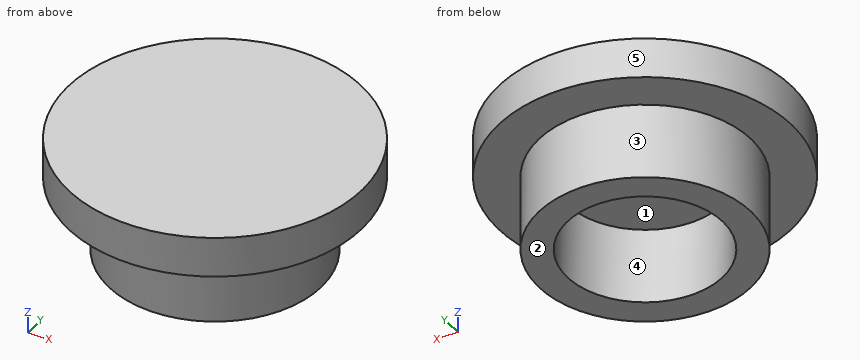
from build123d import *

# Parameters (mm, degrees)
SKETCH1_R           = 9.2075
BOSS_EXTRUDE1_DEPTH = 2.54
SKETCH2_R           = 6.6675
SKETCH2_R_2         = 4.8895
BOSS_EXTRUDE2_DEPTH = 4.7625


with BuildPart() as part:
    # Sketch1 → Boss-Extrude1 (new body)
    with BuildSketch(Plane.XY):
        Circle(SKETCH1_R)
    extrude(amount=BOSS_EXTRUDE1_DEPTH)

    # Sketch2 → Boss-Extrude2 (add)
    with BuildSketch(Plane(origin=(0, 0, 0), x_dir=(-1, 0, 0), z_dir=(0, 0, -1))):
        Circle(SKETCH2_R)
        Circle(SKETCH2_R_2, mode=Mode.SUBTRACT)
    extrude(amount=BOSS_EXTRUDE2_DEPTH)


solid = part.part
Build history of the part. All positions in model axes, mm. Face numbers are marked on the shaded views. A direction names the side the tool comes from. Round coordinates to 2 decimals unless told otherwise and drop trailing zeros. Write each loop counter-clockwise with the first axis right and the second up, starting at its lowest first coordinate (ties: lowest second). Pieces come first, ordered by that corner, then holes. Notation, with made-up numbers: M -26.5,15 L 16.5,15 A8 cw 16.5,19 Z; hole C 74.25,27.5 d4. An arc over 180 degrees is marked long. Answer in a Markdown table with one row per item.
1. Which spindle directions (+Z, -Z, +X, -X, +Y, -Y) get a long thin tool onto all of the face, cutting with end or side? Do the marked faces 4 and 5. Say none if no direction does.
Geometry check:
| item | result |
|---|---|
| face 4 | -Z |
| face 5 | +Z, -Z |
2. Saw through at C-C (y = 3). List the corners of the cut face in (x, z).
Geometry check:
| item | result |
|---|---|
| outline | M -8.71,0 L -5.95,0 L -5.95,-4.76 L -3.86,-4.76 L -3.86,0 L 3.86,0 L 3.86,-4.76 L 5.95,-4.76 L 5.95,0 L 8.71,0 L 8.71,2.54 L -8.71,2.54 Z |
3. Saw through at D-D (z = 1.5). List the corners of the cut face in (x, y) (1 decimal), and give its area (3 significant figures).
Geometry check:
| item | result |
|---|---|
| outline | C 0,0 d18.4 |
| area | 266 mm2 |
4. Mould opens along X. For the marked faces 1, 2 and 3 say: +X half, -X half, draft (parallel to the pull), parting line (faces both ways), or undercut.
Geometry check:
| item | result |
|---|---|
| face 1 | undercut |
| face 2 | draft |
| face 3 | parting line |
5. Saw through at B-B (z = -0.5). List the corners of the cut face in (x, y) (1 decimal), and give its area (3 significant figures).
Geometry check:
| item | result |
|---|---|
| outline | C 0,0 d13.3; hole C 0,0 d9.8 |
| area | 64.6 mm2 |
6. Flat gauge pins, fed straight in: P1, Ø3, axis at x = 7, z = 1, coming from the -Y side; P2, Ø9, axis at x = -4, y = -1.5, coming from the -Z side; P3, Ø3, axis at x = -4, z = 0.5, coming from the +Y side. Where does each tip first touch, or does it go through?
Geometry check:
| item | result |
|---|---|
| P1 | y = -7.38 |
| P2 | z = -4.76 |
| P3 | y = 8.86 |
7. Saw through at A-A (x = 0). List the corners of the cut face in (y, z).
Geometry check:
| item | result |
|---|---|
| outline | M -9.21,0 L -6.67,0 L -6.67,-4.76 L -4.89,-4.76 L -4.89,0 L 4.89,0 L 4.89,-4.76 L 6.67,-4.76 L 6.67,0 L 9.21,0 L 9.21,2.54 L -9.21,2.54 Z |
8. Probe L1, parallel to Y at x = 0, z = -1.2; L2, parallel to Z at x = 7.5, y = 2; L3, parallel to Y at x = 3, z = -1. List the from-to ranges inside material, lowest first. Write a range as [from, to].
Geometry check:
| item | result |
|---|---|
| L1 | [-6.67, -4.89], [4.89, 6.67] |
| L2 | [0, 2.54] |
| L3 | [-5.95, -3.86], [3.86, 5.95] |
